Could you check a few things on this model? Use its own coordinates, in mm. A direction names the side the tool comes from. Round coordinates to 2 decimals unless told otherwise and drop trailing zeros. Write each loop counter-clockwise with the first axis right and the second up, starting at its lowest first coordinate (ties: lowest second). Pieces come first, ordered by that corner, then holes. Notation, with made-up numbers: (31.5, 48.25) -> (53.5, 48.25) arc R29 ccw to (53.5, 86.25) -> close; hole circle Ø1 at (73.5, 73.25). An arc over 180 degrees is marked (long way). Return JSON: item names as keys, results as strings.
Autodesk Inventor part; units mm, degrees
ref_plane "YZ Plane" through (0, 0, 0) normal (1, 0, 0) x (0, 1, 0)
ref_plane "XZ Plane" through (0, 0, 0) normal (0, 1, 0) x (-1, 0, 0)
ref_plane "XY Plane" through (0, 0, 0) normal (0, 0, 1) x (1, 0, 0)
sketch "草图1" plane through (0, 0, 0) normal (0, 0, 1) x (1, 0, 0)
  line L0 (0, 5) -> (61, 5)
  line L1 (61, 5) -> (61, 75)
  line L2 (61, 75) -> (65, 75)
  line L3 (65, 75) -> (65, 0)
  line L4 (65, 0) -> (0, 0)
  line L5 (0, 34.2328) -> (0, -13.4923)
  line L6 (0, 5) -> (-61, 5)
  line L7 (-61, 5) -> (-61, 75)
  line L8 (-65, 75) -> (-65, 0)
  line L9 (-65, 0) -> (0, 0)
  line L10 (-61, 75) -> (-65, 75)
  dimension "d0" = 5
  dimension "d1" = 130
  dimension "d2" = 4
  dimension "d3" = 75
extrude "拉伸1" add sketch "草图1" along normal blind 138
sketch "草图2" plane through (65, 0, 0) normal (1, 0, 0) x (0, 0, -1)
  line L0 (-107.5, 24) -> (-72.5, 24) construction
  line L1 (0, 5) -> (-138, 5)
  circle A0 centre (-72.5, 24) radius 15.5 construction
  circle A1 centre (-107.5, 24) radius 15.5 construction
  circle A2 centre (-57, 24) radius 2.1
  circle A3 centre (-123, 24) radius 2.1
  line L2 (-138, 0) -> (-138, 75)
  circle A4 centre (-115.25, 10.5766) radius 2.1
  circle A5 centre (-99.75, 10.5766) radius 2.1
  circle A6 centre (-92, 24) radius 2.1
  circle A7 centre (-99.75, 37.4234) radius 2.1
  circle A8 centre (-115.25, 37.4234) radius 2.1
  circle A9 centre (-64.75, 37.4234) radius 2.1
  circle A10 centre (-80.25, 37.4234) radius 2.1
  circle A11 centre (-88, 24) radius 2.1
  circle A12 centre (-80.25, 10.5766) radius 2.1
  circle A13 centre (-64.75, 10.5766) radius 2.1
  point P0 (0, 0)
  dimension "d8" = 31
  dimension "d9" = 31
  dimension "d6" = 35
  dimension "d10" = 4.2
  dimension "d11" = 4.2
  dimension "d12" = 15
  dimension "d15" = 360
  dimension "d19" = 360
  dimension "d24" = 19
extrude "拉伸2" cut sketch "草图2" against normal blind 150 contours A2 | A3 | A4 | A5 | A8 | A9 | A12 | A13
sketch "草图3" plane through (65, 0, 0) normal (1, 0, 0) x (0, 0, -1)
  circle A0 centre (-90, 34) radius 3.25
  circle A1 centre (-90, 25) radius 3.25
  circle A2 centre (-90, 16) radius 3.25
  circle A3 centre (-98, 41.2575) radius 3.25
  circle A4 centre (-82, 41.2575) radius 3.25
  point P0 (0, 0)
extrude "拉伸3" cut sketch "草图3" against normal blind 150
sketch "草图4" plane through (0, 0, 0) normal (0, 0, -1) x (-1, 0, 0)
  line L0 (-65, 0) -> (-65, 75)
  line L1 (65, 0) -> (-65, 0)
  line L2 (65, 75) -> (65, 0)
  line L3 (-65, 75) -> (-50, 75)
  line L4 (-50, 75) -> (-50, 15)
  line L5 (-50, 15) -> (50, 15)
  line L6 (50, 15) -> (50, 75)
  line L7 (50, 75) -> (65, 75)
  point P0 (0, 0)
  dimension "d27" = 15
  dimension "d28" = 15
  dimension "d29" = 15
extrude "拉伸4" add sketch "草图4" along normal blind 5
sketch "草图5" plane through (0, 0, 0) normal (0, 0, 1) x (1, 0, 0)
  line L0 (61, 75) -> (61, 5)
  line L1 (50, 75) -> (61, 75)
  line L2 (50, 15) -> (50, 75)
  line L3 (-50, 15) -> (50, 15)
  line L4 (-50, 75) -> (-50, 15)
  line L5 (-61, 75) -> (-50, 75)
  line L6 (-61, 5) -> (-61, 75)
  line L7 (61, 5) -> (-61, 5)
  line L8 (61, 11) -> (55, 5)
  line L9 (0, 97.2027) -> (0, -45.2903)
  line L10 (-61, 11) -> (-55, 5)
  point P0 (0, 0)
  dimension "d32" = 45
  dimension "d33" = 6
extrude "拉伸5" add sketch "草图5" along normal blind 55 contours L0 L7 L8 | L7 L6 L10
chamfer "倒角1" distance 2 angle 45 2 edges at (58, 8, 55) (-58, 8, 55)
sketch "草图7" plane through (0, 0, 138) normal (0, 0, 1) x (1, 0, 0)
  line L0 (-65, 0) -> (65, 0)
  line L1 (65, 0) -> (65, 75)
  line L2 (65, 75) -> (61, 75)
  line L3 (61, 75) -> (61, 5)
  line L4 (61, 5) -> (-61, 5)
  line L5 (-61, 5) -> (-61, 75)
  line L6 (-61, 75) -> (-65, 75)
  line L7 (-65, 75) -> (-65, 0)
  point P0 (0, 0)
extrude "拉伸6" add sketch "草图7" along normal blind 25
sketch "草图13" plane through (-65, 0, -5) normal (-1, 0, 0) x (0, 0, 1)
  line L0 (80, 55) -> (110, 55) construction
  line L1 (110, 55) -> (110, 67) construction
  line L2 (110, 67) -> (80, 67) construction
  line L3 (80, 67) -> (80, 55) construction
  line L4 (80, 55) -> (110, 67) construction
  line L5 (110, 55) -> (80, 67) construction
  line L6 (0, 75) -> (168, 75)
  circle A0 centre (95, 34) radius 3.25
  line L7 (95, 34) -> (95, 46.2012) construction
  circle A1 centre (80, 55) radius 2.1
  circle A2 centre (110, 55) radius 2.1
  circle A3 centre (95, 55) radius 2.1
  circle A4 centre (80, 67) radius 2.1
  circle A5 centre (110, 67) radius 2.1
  point P0 (5, 0)
  point P1 (95, 61)
  point P2 (233, 75)
  dimension "d62" = 8
  dimension "d63" = 30
  dimension "d64" = 20
  dimension "d65" = 4.2
  dimension "d66" = 4.2
  dimension "d67" = 4.2
  dimension "d68" = 4.2
  dimension "d69" = 4.2
extrude "拉伸11" cut sketch "草图13" against normal blind 150 contours A1 | A2 | A3 | A4 | A5
sketch "草图14" plane through (0, 0, 163) normal (0, 0, 1) x (1, 0, 0)
  line L0 (65, 0) -> (65, 75)
  line L1 (65, 75) -> (61, 75)
  line L2 (61, 75) -> (61, 5)
  line L3 (61, 5) -> (-61, 5)
  line L4 (-61, 5) -> (-61, 75)
  line L5 (-61, 75) -> (-65, 75)
  line L6 (-65, 75) -> (-65, 0)
  line L7 (-65, 0) -> (65, 0)
  point P0 (0, 0)
extrude "拉伸12" add sketch "草图14" along normal blind 45
sketch "草图15" plane through (-55, 5, 0) normal (0, 1, 0) x (1, 0, 0)
  line L0 (-6, -55) -> (-6, -208)
  line L1 (116, 0) -> (116, -208)
  line L2 (-6, -208) -> (116, -208)
  line L3 (116, -208) -> (116, -202)
  line L4 (116, -202) -> (-6, -202)
  line L5 (-6, -202) -> (-6, -208)
  point P0 (55, 0)
  point P1 (-6, -202)
  dimension "d74" = 6
extrude "拉伸13" add sketch "草图15" along normal up to surface (70 mm away)
fillet "圆角2" radius 30 1 edges at (0, 5, 202)
fillet "圆角3" radius 35 1 edges at (0, 0, 208)
properties part number "车架"
1) For faces 1 (the face through (63.028, 16.143, 93.247)), 2 (the face through (58, 8, 26)), which set-ups out of +Z, -Z, +X, -X, +Y, -Y let a thin tool reach every point of the face, with its end or its side?
Return value:
{"face 1": "+X, -X", "face 2": "+Y"}
2) I want a section at A-A, the plane z = 105. Please give me the cut outline in (x, y).
Return value:
{"outline": "(-65, 0) -> (65, 0) -> (65, 52.9) -> (61, 52.9) -> (61, 5) -> (-61, 5) -> (-61, 52.9) -> (-65, 52.9) -> close; (-65, 57.1) -> (-61, 57.1) -> (-61, 64.9) -> (-65, 64.9) -> close; (-65, 69.1) -> (-61, 69.1) -> (-61, 75) -> (-65, 75) -> close; (61, 57.1) -> (65, 57.1) -> (65, 64.9) -> (61, 64.9) -> close; (61, 69.1) -> (65, 69.1) -> (65, 75) -> (61, 75) -> close"}
3) Will these pins go through, and if not, where does the flat tip stop? pin 1 Ø4 at (y, z) = (55, 105) entering from -X; pin 2 Ø10 at (x, z) = (14, 80.5) entering from +Y; pin 3 Ø2.5 at (x, y) = (58.5, 6) entering from +Z; pin 4 Ø5 at (x, y) = (-26.5, 12) entering from +Z.
Return value:
{"pin 1": "through", "pin 2": "y = 5", "pin 3": "z = 194.33", "pin 4": "z = 201.37"}
4) If I drill on probe 1 along Y at (x, z) = (63, 115); probe 2 along Y at (x, z) = (62.4, 90); probe 3 along Y at (x, z) = (-63.3, 105), over which ranges is the centre line in solid material (lowest first)? Write a range as [from, to].
Return value:
{"probe 1": "[0, 8.49], [12.66, 35.34], [39.51, 75]", "probe 2": "[0, 12.75], [19.25, 21.75], [28.25, 30.75], [37.25, 52.9], [57.1, 75]", "probe 3": "[0, 52.9], [57.1, 64.9], [69.1, 75]"}
5) I want a section at B-B, the plane y = 67. Please give me the cut outline in (x, z).
Return value:
{"outline": "(-65, -5) -> (-50, -5) -> (-50, 0) -> (-61, 0) -> (-61, 72.9) -> (-65, 72.9) -> close; (-65, 77.1) -> (-61, 77.1) -> (-61, 102.9) -> (-65, 102.9) -> close; (-65, 107.1) -> (-61, 107.1) -> (-61, 202) -> (61, 202) -> (61, 107.1) -> (65, 107.1) -> (65, 208) -> (-65, 208) -> close; (50, -5) -> (65, -5) -> (65, 72.9) -> (61, 72.9) -> (61, 0) -> (50, 0) -> close; (61, 77.1) -> (65, 77.1) -> (65, 102.9) -> (61, 102.9) -> close"}
6) Thinking about a two-plate mould opening in X: for faces 3 (the face through (62.972, 53.722, 73.334)), 4 (the face through (-61, 47, 100)), 5 (the face through (-65, 38, 100)), which applies, pulls with the +X half, pulls with the -X half, needs draft (parallel to the pull), parting line crosses it, or undercut?
Return value:
{"face 3": "needs draft", "face 4": "undercut", "face 5": "pulls with the -X half"}
7) I want a section at C-C, the plane x = -25. Please give me the cut outline in (y, z).
Return value:
{"outline": "(0, -5) -> (15, -5) -> (15, 0) -> (5, 0) -> (5, 172) arc R30 cw to (35, 202) -> (75, 202) -> (75, 208) -> (35, 208) arc R35 ccw to (0, 173) -> close"}
8) I want a section at D-D, the plane y = 48.5. Please give me the cut outline in (x, z).
Return value:
{"outline": "(-65, -5) -> (-50, -5) -> (-50, 0) -> (-61, 0) -> (-61, 202) -> (61, 202) -> (61, 0) -> (50, 0) -> (50, -5) -> (65, -5) -> (65, 208) -> (-65, 208) -> close"}
